```python
from build123d import *

# Parameters (mm, degrees)
SKETCH_1_R          = 25
SKETCH_1_W          = 3
SKETCH_1_H          = 10
SKETCH_1_R_2        = 2
SKETCH_1_R_3        = 1.5
SKETCH_1_R_4        = 2.75
EXTRUDE_1_DEPTH     = 5
CUT_EXTRUDE_START   = -10
SKETCH_3_W          = 3.5
SKETCH_3_H          = 10.5
SKETCH_3_W_2        = 3
SKETCH_3_H_2        = 10
CUT_EXTRUDE_1_DEPTH = 10


with BuildPart() as part:
    # 草图1 → 凸台-拉伸1 (new body)
    with BuildSketch(Plane.XY):
        Circle(SKETCH_1_R)
        with Locations((11.5, 0)):
            Rectangle(SKETCH_1_W, SKETCH_1_H, mode=Mode.SUBTRACT)
        with Locations((-10, -17.320508076)):
            Circle(SKETCH_1_R_2, mode=Mode.SUBTRACT)
        with Locations((-7.071067812, -7.071067812)):
            Circle(SKETCH_1_R_3, mode=Mode.SUBTRACT)
        with BuildLine():
            Line((-10, -1.322875656), (-10, -5))
            Line((-10, -5), (-13, -5))
            Line((-13, -5), (-13, -1.322875656))
            ThreePointArc((-13, -1.322875656), (-13.5, 0), (-13, 1.322875656))
            Line((-13, 1.322875656), (-13, 5))
            Line((-13, 5), (-10, 5))
            Line((-10, 5), (-10, 1.322875656))
            ThreePointArc((-10, 1.322875656), (-9.5, 0), (-10, -1.322875656))
        make_face(mode=Mode.SUBTRACT)
        with Locations((10, -17.320508076)):
            Circle(SKETCH_1_R_2, mode=Mode.SUBTRACT)
        with BuildLine():
            Line((1.322875656, -10), (5, -10))
            Line((5, -10), (5, -13))
            Line((5, -13), (1.322875656, -13))
            ThreePointArc((1.322875656, -13), (0, -13.5), (-1.322875656, -13))
            Line((-1.322875656, -13), (-5, -13))
            Line((-5, -13), (-5, -10))
            Line((-5, -10), (-1.322875656, -10))
            ThreePointArc((-1.322875656, -10), (0, -9.5), (1.322875656, -10))
        make_face(mode=Mode.SUBTRACT)
        with Locations((7.071067812, -7.071067812)):
            Circle(SKETCH_1_R_3, mode=Mode.SUBTRACT)
        with Locations((-20, 0)):
            Circle(SKETCH_1_R_2, mode=Mode.SUBTRACT)
        with Locations((-7.071067812, 7.071067812)):
            Circle(SKETCH_1_R_3, mode=Mode.SUBTRACT)
        with BuildLine():
            Line((-1.322875656, 10), (-5, 10))
            Line((-5, 10), (-5, 13))
            Line((-5, 13), (-1.322875656, 13))
            ThreePointArc((-1.322875656, 13), (0, 13.5), (1.322875656, 13))
            Line((1.322875656, 13), (5, 13))
            Line((5, 13), (5, 10))
            Line((5, 10), (1.322875656, 10))
            ThreePointArc((1.322875656, 10), (0, 9.5), (-1.322875656, 10))
        make_face(mode=Mode.SUBTRACT)
        with Locations((-10, 17.320508076)):
            Circle(SKETCH_1_R_2, mode=Mode.SUBTRACT)
        Circle(SKETCH_1_R_4, mode=Mode.SUBTRACT)
        with Locations((10, 17.320508076)):
            Circle(SKETCH_1_R_2, mode=Mode.SUBTRACT)
        with Locations((7.071067812, 7.071067812)):
            Circle(SKETCH_1_R_3, mode=Mode.SUBTRACT)
        with Locations((20, 0)):
            Circle(SKETCH_1_R_2, mode=Mode.SUBTRACT)
    extrude(amount=EXTRUDE_1_DEPTH)

    # 草图3 → 切除-拉伸1 (cut)
    # profile 1 of 4: a face of its own
    with BuildSketch(Plane.XY.offset(5).offset(CUT_EXTRUDE_START)):
        with BuildLine():
            Line((-5.25, 9.75), (-5.25, 13.25))
            Line((-5.25, 13.25), (-1.414213562, 13.25))
            ThreePointArc((-1.414213562, 13.25), (0, 13.75), (1.414213562, 13.25))
            Line((1.414213562, 13.25), (5.25, 13.25))
            Line((5.25, 13.25), (5.25, 9.75))
            Line((5.25, 9.75), (1.414213562, 9.75))
            ThreePointArc((1.414213562, 9.75), (0, 9.25), (-1.414213562, 9.75))
            Line((-1.414213562, 9.75), (-5.25, 9.75))
        make_face()
        with BuildLine():
            Line((-5, 10), (-5, 13))
            Line((-5, 13), (-1.322875656, 13))
            ThreePointArc((-1.322875656, 13), (0, 13.5), (1.322875656, 13))
            Line((1.322875656, 13), (5, 13))
            Line((5, 13), (5, 10))
            Line((5, 10), (1.322875656, 10))
            ThreePointArc((1.322875656, 10), (0, 9.5), (-1.322875656, 10))
            Line((-1.322875656, 10), (-5, 10))
        make_face(mode=Mode.SUBTRACT)
    # profile 2 of 4: a face of its own
    with BuildSketch(Plane.XY.offset(5).offset(CUT_EXTRUDE_START)):
        with BuildLine():
            Line((-13.25, -5.25), (-13.25, -1.414213562))
            ThreePointArc((-13.25, -1.414213562), (-13.75, 0), (-13.25, 1.414213562))
            Line((-13.25, 1.414213562), (-13.25, 5.25))
            Line((-13.25, 5.25), (-9.75, 5.25))
            Line((-9.75, 5.25), (-9.75, 1.414213562))
            ThreePointArc((-9.75, 1.414213562), (-9.25, 0), (-9.75, -1.414213562))
            Line((-9.75, -1.414213562), (-9.75, -5.25))
            Line((-9.75, -5.25), (-13.25, -5.25))
        make_face()
        with BuildLine():
            Line((-13, -5), (-13, -1.322875656))
            ThreePointArc((-13, -1.322875656), (-13.5, 0), (-13, 1.322875656))
            Line((-13, 1.322875656), (-13, 5))
            Line((-13, 5), (-10, 5))
            Line((-10, 5), (-10, 1.322875656))
            ThreePointArc((-10, 1.322875656), (-9.5, 0), (-10, -1.322875656))
            Line((-10, -1.322875656), (-10, -5))
            Line((-10, -5), (-13, -5))
        make_face(mode=Mode.SUBTRACT)
    # profile 3 of 4: a face of its own
    with BuildSketch(Plane.XY.offset(5).offset(CUT_EXTRUDE_START)):
        with BuildLine():
            Line((5.25, -9.75), (1.414213562, -9.75))
            ThreePointArc((1.414213562, -9.75), (0, -9.25), (-1.414213562, -9.75))
            Line((-1.414213562, -9.75), (-5.25, -9.75))
            Line((-5.25, -9.75), (-5.25, -13.25))
            Line((-5.25, -13.25), (-1.414213562, -13.25))
            ThreePointArc((-1.414213562, -13.25), (0, -13.75), (1.414213562, -13.25))
            Line((1.414213562, -13.25), (5.25, -13.25))
            Line((5.25, -13.25), (5.25, -9.75))
        make_face()
        with BuildLine():
            Line((5, -10), (1.322875656, -10))
            ThreePointArc((1.322875656, -10), (0, -9.5), (-1.322875656, -10))
            Line((-1.322875656, -10), (-5, -10))
            Line((-5, -10), (-5, -13))
            Line((-5, -13), (-1.322875656, -13))
            ThreePointArc((-1.322875656, -13), (0, -13.5), (1.322875656, -13))
            Line((1.322875656, -13), (5, -13))
            Line((5, -13), (5, -10))
        make_face(mode=Mode.SUBTRACT)
    # profile 4 of 4: a face of its own
    with BuildSketch(Plane.XY.offset(5).offset(CUT_EXTRUDE_START)):
        with Locations((11.5, 0)):
            Rectangle(SKETCH_3_W, SKETCH_3_H)
        with Locations((11.5, 0)):
            Rectangle(SKETCH_3_W_2, SKETCH_3_H_2, mode=Mode.SUBTRACT)
    extrude(amount=CUT_EXTRUDE_1_DEPTH, mode=Mode.SUBTRACT)


solid = part.part
```
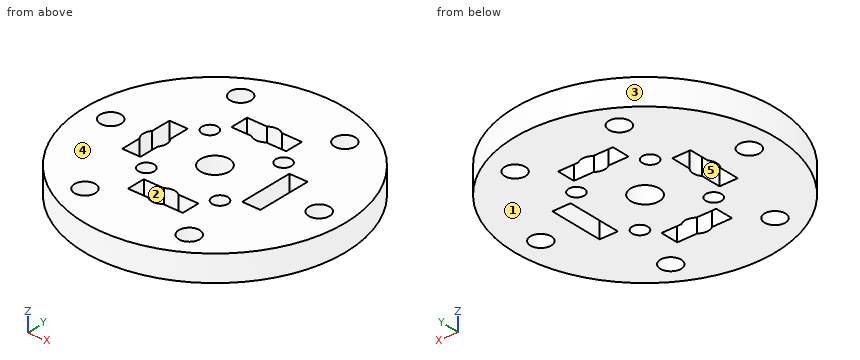
Build history of the part. All positions in model axes, mm. Face numbers are marked on the shaded views. A direction names the side the tool comes from. Round coordinates to 2 decimals unless told otherwise and drop trailing zeros. Loops run counter-clockwise (first coordinate to the right, second up) from the corner with the lowest first, then second, coordinate; pieces in that order, holes last.
Item 1: Saw through at B-B (y = 0). List the corners of the cut face in (x, z).
Item 2: Which spindle directions (+Z, -Z, +X, -X, +Y, -Y) get a long thin tool onto all of the face, cutting with end or side? Do the marked faces 4 and 5. Say none if no direction does.
Item 3: Saw through at C-C (x = 0). List the corners of the cut face in (y, z).
Item 4: Saw through at A-A (x = 20). List the corners of the cut face in (y, z), then the cut area to 3 significant figures.
Item 5: Two-plate mould, pull along X, no slides. Class the marked faces 1, 2 and 3: released by +X, released by -X, zero draft, split by the parting line, or undercut.
Item 6: Saw through at D-D (z = 3). State how many separate pieces and enclosed holes the cut face has, then the cut area to 3 significant figures.
Item 7: Pin check, flat tips, straight feed: P1, Ø1, axis at y = 12.5, z = 1.5, coming from the +X side; P2, Ø1, axis at x = -10.5, z = 2.5, coming from the -Y side; P3, Ø1.5, axis at y = 7.5, z = 1.5, coming from the +X side; P4, Ø5, axis at x = -10, y = 17.32, coming from the +Z side. Stop position of each tip, or through.
Item 8: Drill centre lines: line 1 along X through (y, z) = (6, 4.2); line 2 along X through (y, z) = (-1.5, 4.55); line 3 along Y through (x, z) = (-10, 2.25). Where is each one in solid material? Low to high.
Worked answers:
1. outline: (-25, 0) - (-22, 0) - (-22, 5) - (-25, 5) - close; (-18, 0) - (-13.75, 0) - (-13.75, 5) - (-18, 5) - close; (-9.25, 0) - (-2.75, 0) - (-2.75, 5) - (-9.25, 5) - close; (2.75, 0) - (9.75, 0) - (9.75, 5) - (2.75, 5) - close; (13.25, 0) - (18, 0) - (18, 5) - (13.25, 5) - close; (22, 0) - (25, 0) - (25, 5) - (22, 5) - close
2. face 4: +Z, +X, -X, +Y, -Y
2. face 5: +Z, -Z
3. outline: (-25, 0) - (-13.75, 0) - (-13.75, 5) - (-25, 5) - close; (-9.25, 0) - (-2.75, 0) - (-2.75, 5) - (-9.25, 5) - close; (2.75, 0) - (9.25, 0) - (9.25, 5) - (2.75, 5) - close; (13.75, 0) - (25, 0) - (25, 5) - (13.75, 5) - close
4. outline: (-15, 0) - (-2, 0) - (-2, 5) - (-15, 5) - close; (2, 0) - (15, 0) - (15, 5) - (2, 5) - close
4. area: 130 mm2
5. face 1: zero draft
5. face 2: undercut
5. face 3: split by the parting line
6. separate pieces: 1
6. enclosed holes: 15
6. area: 1,680 mm2
7. P1: stops at x = 21.93
7. P2: stops at y = -22.91
7. P3: stops at x = 24.07
7. P4: stops at z = 5
8. line 1: x = -24.27 to -8.12, -6.02 to 6.02, 8.12 to 24.27
8. line 2: x = -24.95 to -21.32, -18.68 to -13.25, -9.75 to -2.3, 2.3 to 9.75, 13.25 to 18.68, 21.32 to 24.95
8. line 3: y = -22.91 to -19.32, -15.32 to -5.25, 5.25 to 15.32, 19.32 to 22.91
